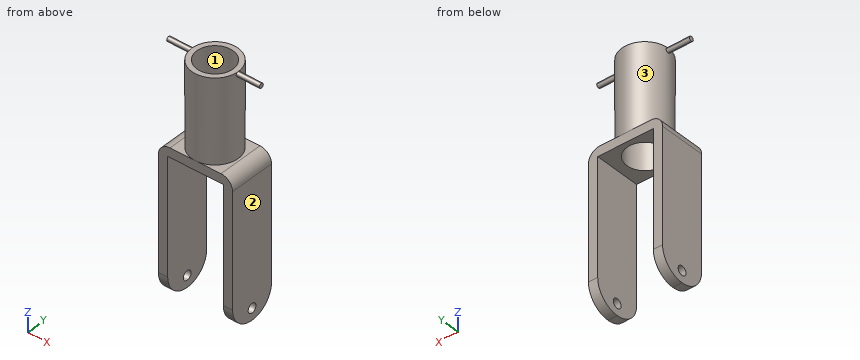
```python
from build123d import *

# Parameters (mm, degrees)
F0_R      = 6.35
F0_R_2    = 0.635
F1_DEPTH  = 63.5
F3_DEPTH  = 1.27
F4_R      = 0.6349
F5_R      = 0.635
F6_DEPTH  = 40.64
F7_R      = 1.27
F8_DEPTH  = 25.4
F9_W      = 15.24
F9_H      = 38.1
F10_DEPTH = 12.7
F11_R     = 4.953
F11_R_2   = 0.635
F12_DEPTH = 25.4
F13_R     = 6.34999
F14_R     = 3.175


# Not quite as in the source:
# - a fillet or chamfer is up to 0.001 mm smaller than in the source, because OpenCascade refuses the exact size


with BuildPart() as f1:
    # F0 (on Top) → F1 (new body)
    with BuildSketch(Plane.XY):
        Circle(F0_R)
        Circle(F0_R_2, mode=Mode.SUBTRACT)
    extrude(amount=F1_DEPTH)

    # F2 (on face) → F3 (join)
    with BuildSketch(Plane.XY.offset(63.5)):
        with BuildLine():
            Line((6.3181702256, -0.635), (12.7, -0.635))
            Line((12.7, -0.635), (12.7, 0.635))
            Line((12.7, 0.635), (6.3181702256, 0.635))
            ThreePointArc((6.3181702256, 0.635), (6.3420375643, 0.3178986216), (6.35, 0))
            ThreePointArc((6.35, 0), (6.3420375643, -0.3178986216), (6.3181702256, -0.635))
        make_face()
        with BuildLine():
            Line((-12.7, -0.635), (-6.3181702256, -0.635))
            ThreePointArc((-6.3181702256, -0.635), (-6.35, 0), (-6.3181702256, 0.635))
            Line((-6.3181702256, 0.635), (-12.7, 0.635))
            Line((-12.7, 0.635), (-12.7, -0.635))
        make_face()
    extrude(amount=-F3_DEPTH)

    # F4 (radius 0.635 in the source; OpenCascade refuses exactly that, so slightly less here)
    f4_edges = [f1.edges().sort_by_distance(p)[0] for p in [
        (9.509085, 0.635, 63.5),
        (9.509085, -0.635, 63.5),
        (-9.509085, 0.635, 63.5),
        (-9.509085, -0.635, 63.5),
        (9.509085, 0.635, 62.23),
        (9.509085, -0.635, 62.23),
        (-9.509085, -0.635, 62.23),
        (-9.509085, 0.635, 62.23),
    ]]
    fillet(f4_edges, radius=F4_R)

    # F5 (on face) → F6 (join)
    with BuildSketch(Plane(origin=(0, 0, 0), x_dir=(1, 0, 0), z_dir=(0, 0, -1))):
        with BuildLine():
            ThreePointArc((0, -6.35), (-6.35, 0), (0, 6.35))
            Line((0, 6.35), (-10.16, 6.35))
            Line((-10.16, 6.35), (-10.16, -6.35))
            Line((-10.16, -6.35), (0, -6.35))
        make_face()
        with BuildLine():
            Line((10.16, -6.35), (10.16, 6.35))
            Line((10.16, 6.35), (0, 6.35))
            ThreePointArc((0, 6.35), (4.4901280605, 4.4901280605), (6.35, 0))
            ThreePointArc((6.35, 0), (4.4901280605, -4.4901280605), (0, -6.35))
            Line((0, -6.35), (10.16, -6.35))
        make_face()
        Circle(F5_R)
    extrude(amount=-F6_DEPTH)

    # F7 (on face) → F8 (cut)
    with BuildSketch(Plane(origin=(-10.16, 0, 0), x_dir=(0, -1, 0), z_dir=(-1, 0, 0))):
        with Locations((0, 3.175)):
            Circle(F7_R)
    extrude(amount=-F8_DEPTH, mode=Mode.SUBTRACT)

    # F9 (on face) → F10 (cut)
    with BuildSketch(Plane.XZ.offset(6.35)):
        with Locations((0, 19.05)):
            Rectangle(F9_W, F9_H)
    extrude(amount=-F10_DEPTH, mode=Mode.SUBTRACT)

    # F11 (on face) → F12 (cut, through all)
    with BuildSketch(Plane.XY.offset(63.5)):
        Circle(F11_R)
        Circle(F11_R_2, mode=Mode.SUBTRACT)
        Circle(F11_R_2)
    extrude(amount=-F12_DEPTH, mode=Mode.SUBTRACT)

    # F13 (radius 6.35 in the source; OpenCascade refuses exactly that, so slightly less here)
    f13_edges = [f1.edges().sort_by_distance(p)[0] for p in [
        (8.89, 6.35, 0),
        (8.89, -6.35, 0),
        (-8.89, -6.35, 0),
        (-8.89, 6.35, 0),
    ]]
    fillet(f13_edges, radius=F13_R)

    # F14
    f14_edges = [f1.edges().sort_by_distance(p)[0] for p in [
        (10.16, 0, 40.64),
        (-10.16, 0, 40.64),
    ]]
    fillet(f14_edges, radius=F14_R)


solid = f1.part
```
Geometry: final body of the model. Coordinates: model frame, mm. Face numbers are marked on the shaded views. Round coordinates to 2 decimals unless told otherwise and drop trailing zeros. Order: outer loops, then holes, each group sorted by start corner. A loop starts at its lowest first (then second) coordinate and runs counter-clockwise, first axis right, second up. Notation, with made-up numbers: (6, 17) -> (61, 17) arc R33 ccw to (61, 45) -> close; hole circle Ø4 at (75.25, 71.5). An arc over 180 degrees is marked (long way). Use CSV: the item, a comma, the result in double quotes. Start each with the question number.
1) Section B-B (x = 1.5). Return the cut outline in (y, z).
2) Draft query along X for the marked faces 1, 2 and 3. Return one class per face: +X half, -X half, draft (parallel to the pull), parting line (faces both ways), or undercut.
3) Material intervals for line 1 along X through (y, z) = (2.5, 10); line 2 along Z through (x, y) = (-9.05, 0) (3 decimals); line 3 along Y through (x, z) = (0, 45.75), sorted ascending. Write a range as from..to.
4) Section D-D (z = 53.5). Return the cut outline in (x, y), and give its area (3 significant figures).
5) Section A-A (z = 16). Return the cut outline in (x, y), and give its area (3 significant figures).
6) Section C-C (y = -3.5). Return the cut outline in (x, z) (3 decimals).
7) First-contact query: pin 1 Ø10 at (x, z) = (3.5, 34) entering from -Y; pin 2 Ø3.5 at (x, y) = (-3, 0) entering from +Z; pin 3 Ø4 at (y, z) = (1, 11.5) entering from +X; pin 4 Ø6.5 at (y, z) = (3, 16.5) entering from -X. Flat tips, straight axial feed; report the tip coordinate or a pass-through.
Returned:
1,outline,"(-6.35, 38.1) -> (-4.72, 38.1) -> (-4.72, 63.5) -> (-6.17, 63.5) -> (-6.17, 40.64) -> (-6.35, 40.64) -> close; (4.72, 38.1) -> (6.35, 38.1) -> (6.35, 40.64) -> (6.17, 40.64) -> (6.17, 63.5) -> (4.72, 63.5) -> close"
2,face 1,"undercut"
2,face 2,"+X half"
2,face 3,"parting line"
3,line 1,"x = -10.16..-7.62, 7.62..10.16"
3,line 2,"z = 0..1.905, 4.445..39.877, 62.23..63.5"
3,line 3,"y = -6.35..-4.95, 4.95..6.35"
4,outline,"circle Ø12.7 at (0, 0); hole circle Ø9.91 at (0, 0)"
4,area,"49.6 mm²"
5,outline,"(-10.16, -6.35) -> (-7.62, -6.35) -> (-7.62, 6.35) -> (-10.16, 6.35) -> close; (7.62, -6.35) -> (10.16, -6.35) -> (10.16, 6.35) -> (7.62, 6.35) -> close"
5,area,"64.5 mm²"
6,outline,"(-10.16, 1.052) -> (-7.62, 1.052) -> (-7.62, 38.1) -> (-3.505, 38.1) -> (-3.505, 63.5) -> (-5.298, 63.5) -> (-5.298, 40.64) -> (-6.985, 40.64) arc R3.175 ccw to (-10.16, 37.465) -> close; (3.505, 38.1) -> (7.62, 38.1) -> (7.62, 1.052) -> (10.16, 1.052) -> (10.16, 37.465) arc R3.175 ccw to (6.985, 40.64) -> (5.298, 40.64) -> (5.298, 63.5) -> (3.505, 63.5) -> close"
7,pin 1,"stops at y = -6.35"
7,pin 2,"passes through"
7,pin 3,"stops at x = 10.16"
7,pin 4,"stops at x = -10.16"
